Could you check a few things on this model? Use its own coordinates, in mm. Give positions to 0.01 mm unless a question says otherwise; leave off trailing zeros. Order: outer loops, then holes, each group sorted by start corner. A loop starts at its lowest first (then second) coordinate and runs counter-clockwise, first axis right, second up. Notation, with made-up numbers: (-20.75, -16) -> (29.25, -16) arc R24 ccw to (29.25, 23) -> close; hole circle Ø10 at (7.25, -5.75). An arc over 180 degrees is marked (long way). One line per item, written item: value.
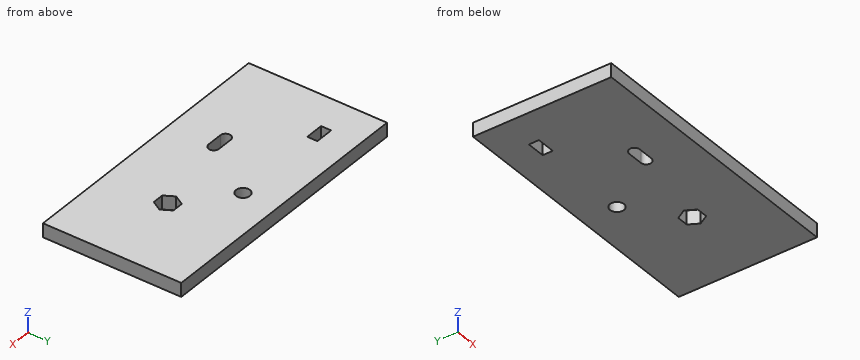
```python
from build123d import *

# Parameters (mm, degrees)
SKETCH1_W           = 200
SKETCH1_H           = 100
BOSS_EXTRUDE1_DEPTH = 10
SKETCH2_R           = 5.053404716
SKETCH2_W           = 13.415300493
SKETCH2_H           = 7.29092418
CUT_EXTRUDE1_DEPTH  = 10


with BuildPart() as part:
    # Sketch1 → Boss-Extrude1 (new body)
    with BuildSketch(Plane.XY):
        with Locations((-100, 50)):
            Rectangle(SKETCH1_W, SKETCH1_H)
    extrude(amount=BOSS_EXTRUDE1_DEPTH)

    # Sketch2 → Cut-Extrude1 (cut)
    with BuildSketch(Plane.XY.offset(10)):
        with Locations((-93.667207309, 74.96711448)):
            Circle(SKETCH2_R)
        with Locations((-167.742996984, 74.96711448)):
            Rectangle(SKETCH2_W, SKETCH2_H)
        with BuildLine():
            Line((-132.163286982, 37.491764192), (-120.789445261, 37.491764192))
            ThreePointArc((-120.789445261, 37.491764192), (-116.998164687, 33.700483618), (-120.789445261, 29.909203044))
            Line((-120.789445261, 29.909203044), (-132.163286982, 29.909203044))
            ThreePointArc((-132.163286982, 29.909203044), (-135.954567556, 33.700483618), (-132.163286982, 37.491764192))
        make_face()
        Polygon((-51.379847062, 45.949236241), (-55.462764603, 53.021056866), (-63.628599685, 53.021056866), (-67.711517226, 45.949236241), (-63.628599685, 38.877415617), (-55.462764603, 38.877415617), align=None)
    extrude(amount=-CUT_EXTRUDE1_DEPTH, mode=Mode.SUBTRACT)


solid = part.part
```
1) Suppose I cut it at A-A, the plane x = -125.5. Write out the boundary of the cut face in (y, z), then the cut area to 3 significant figures.
Answer below:
outline: (0, 0) -> (29.91, 0) -> (29.91, 10) -> (0, 10) -> close; (37.49, 0) -> (100, 0) -> (100, 10) -> (37.49, 10) -> close
area: 924 mm2
2) Suppose I cut it at B-B, the plane y = 44. Write out the boundary of the cut face in (x, z), then the cut area to 3 significant figures.
Answer below:
outline: (-200, 0) -> (-66.59, 0) -> (-66.59, 10) -> (-200, 10) -> close; (-52.51, 0) -> (0, 0) -> (0, 10) -> (-52.51, 10) -> close
area: 1,860 mm2
3) If I drill on line 1 along Y through (x, z) = (-57, 0.75); line 2 along X through (y, z) = (78, 8.5); line 3 along X through (y, z) = (35.5, 6), over which ranges is the centre line in solid material (lowest first)?
Answer below:
line 1: y = 0 to 38.88, 53.02 to 100
line 2: x = -200 to -174.45, -161.04 to -97.71, -89.63 to 0
line 3: x = -200 to -135.5, -117.45 to 0
4) For P1, Ø3, axis at x = -168.5, z = 3.5, coming from the -Y side, with a flat end and sliding along its axis, tell me the tip position at first contact or that it passes through.
Answer below:
P1: stops at y = 0
5) Suppose I cut it at C-C, the plane z = 3. Write out the boundary of the cut face in (x, y), then the cut area to 3 significant figures.
Answer below:
outline: (-200, 0) -> (0, 0) -> (0, 100) -> (-200, 100) -> close; hole (-174.45, 71.32) -> (-161.04, 71.32) -> (-161.04, 78.61) -> (-174.45, 78.61) -> close; hole (-132.16, 29.91) -> (-120.79, 29.91) arc R3.79 ccw to (-120.79, 37.49) -> (-132.16, 37.49) arc R3.79 ccw to start; hole circle Ø10.11 at (-93.67, 74.97); hole (-67.71, 45.95) -> (-63.63, 38.88) -> (-55.46, 38.88) -> (-51.38, 45.95) -> (-55.46, 53.02) -> (-63.63, 53.02) -> close
area: 19,500 mm2
